from build123d import *

# Parameters (mm, degrees)
F0_W     = 270.5
F0_H     = 134
F1_DEPTH = 100
F2_W     = 124
F2_H     = 10
F3_DEPTH = 270.501
F4_W     = 260.5
F4_H     = 10
F5_DEPTH = 134.001


with BuildPart() as f1:
    # F0 (on Top) → F1 (new body)
    with BuildSketch(Plane.XY):
        Rectangle(F0_W, F0_H)
    extrude(amount=F1_DEPTH)

    # F2 (on face) → F3 (cut, through all)
    with BuildSketch(Plane(origin=(-135.25, 0, 0), x_dir=(0, -1, 0), z_dir=(-1, 0, 0))):
        with Locations((0, 90)):
            Rectangle(F2_W, F2_H)
    extrude(amount=-F3_DEPTH, mode=Mode.SUBTRACT)

    # F4 (on face) → F5 (cut, through all)
    with BuildSketch(Plane(origin=(0, 67, 0), x_dir=(-1, 0, 0), z_dir=(0, 1, 0))):
        with Locations((0, 90)):
            Rectangle(F4_W, F4_H)
    extrude(amount=-F5_DEPTH, mode=Mode.SUBTRACT)


solid = f1.part
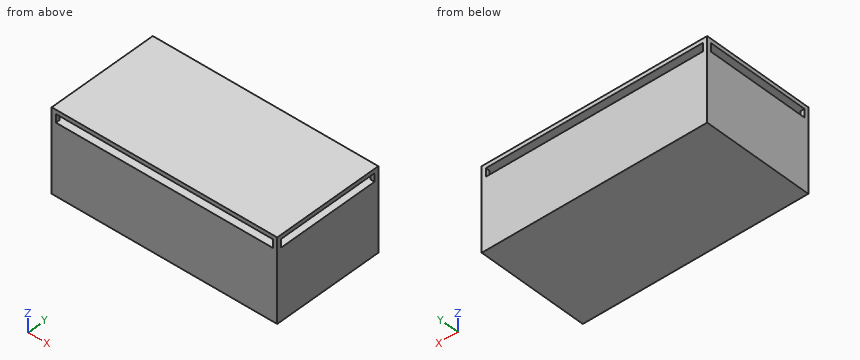
Model file for the job. Use its own axes, mm. Round coordinates to 2 decimals unless told otherwise and drop trailing zeros. Order: outer loops, then holes, each group sorted by start corner. A loop starts at its lowest first (then second) coordinate and runs counter-clockwise, first axis right, second up. Notation, with made-up numbers: M 7.25,-26 L 30.25,-26 A22 cw 30.25,-19 Z; hole C 35,68 d7. An arc over 180 degrees is marked long. Write each question's results on one line, items separated by ' | '. Start each with the question number.
(1) Probe probe 1 along Z at (x, y) = (100, 8). List the from-to ranges inside material, lowest first. Write a range as from..to.
(2) Saw through at A-A, the plane y = 23. Give the cut face in (x, z), then the cut area to 3 significant figures.
(3) Saw through at C-C, the plane x = -24. Give the cut face in (y, z), then the cut area to 3 significant figures.
(4) Saw through at B-B, the plane z = 89. Give the cut face in (x, y).
Established:
1) probe 1: z = 0..85, 95..100
2) outline: M -135.25,0 L 135.25,0 L 135.25,85 L -135.25,85 Z; M -135.25,95 L 135.25,95 L 135.25,100 L -135.25,100 Z | area: 24,300 mm^2
3) outline: M -67,0 L 67,0 L 67,85 L -67,85 Z; M -67,95 L 67,95 L 67,100 L -67,100 Z | area: 12,100 mm^2
4) outline: M -135.25,-67 L -130.25,-67 L -130.25,-62 L -135.25,-62 Z; M -135.25,62 L -130.25,62 L -130.25,67 L -135.25,67 Z; M 130.25,-67 L 135.25,-67 L 135.25,-62 L 130.25,-62 Z; M 130.25,62 L 135.25,62 L 135.25,67 L 130.25,67 Z
